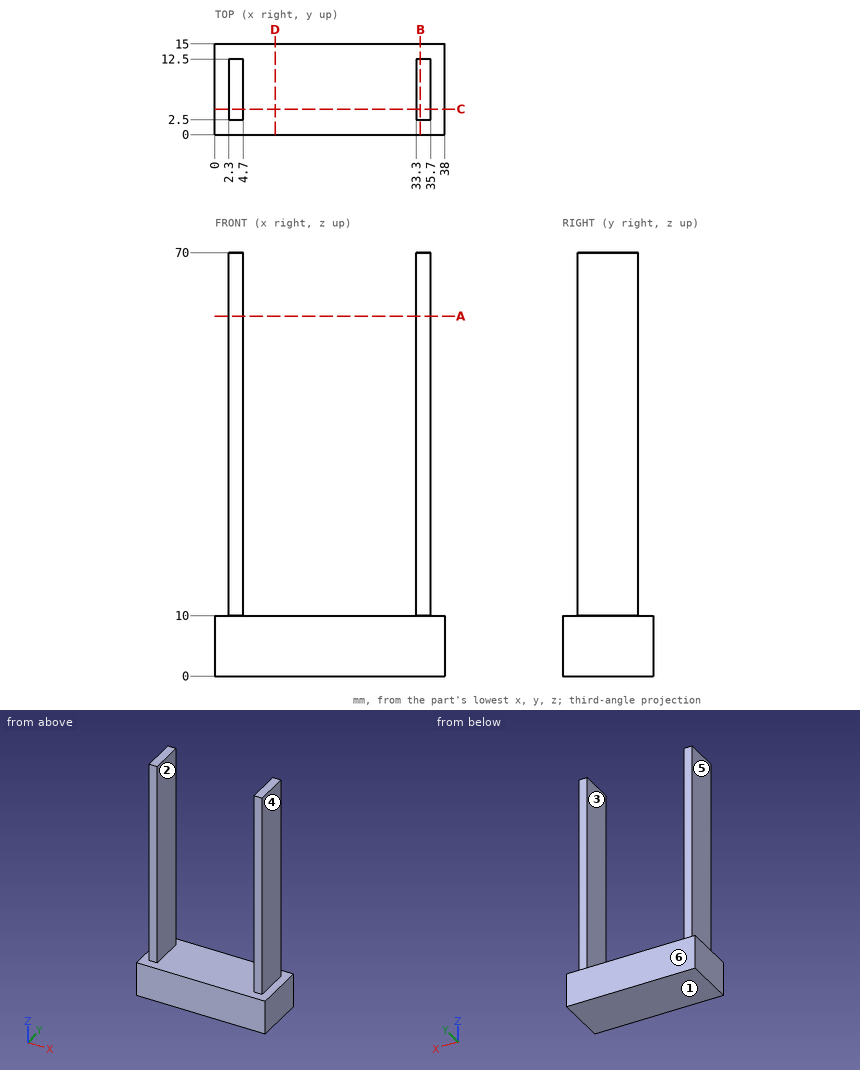
For this review, use the dimensioned drawing (mm, ordinates from the lowest corner) and the shaded views. A direction names the side the tool comes from. Give positions to 0.01 mm unless a question says otherwise; leave off trailing zeros. Order: outer loops, then holes, each group sorted by start corner. A loop starts at its lowest first (then second) coordinate and runs counter-clockwise, first axis right, second up. Notation, with made-up numbers: M 79.25,-15 L 111.25,-15 A10 ccw 111.25,-7 Z; hole C 58,-12 d8. An arc over 180 degrees is marked long. Use one line per item in the form item = value. Start each with the question number.
Item 1: The part is to be moulded in two halves that separate along X. For the marked faces 1, 2, 3 and 4, say which applies: pulls with the +X half, pulls with the -X half, needs draft (parallel to the pull), parting line crosses it, or undercut.
Item 2: For the marked faces 5 and 6, list the 3-axis set-ups (+Z, -Z, +X, -X, +Y, -Y) from which the entire face can be reached by the end or side of a thin tool; tool diameter is ignored.
Item 3: We need section C-C on y = 4.25. Give the boundary of the cut face in (x, z), plus the area to 3 significant figures.
Item 4: We need section A-A on z = 59.5. Give the boundary of the cut face in (x, y).
Item 5: We need section D-D on x = 10. Give the boundary of the cut face in (y, z).
Item 6: We need section B-B on x = 34. Give the boundary of the cut face in (y, z), plus the area to 3 significant figures.
Item 7: To check wall thickness, follow line 1 along X through (y, z) = (8.75, 62); line 2 along Z through (x, y) = (23, 9.5); line 3 along Y through (x, z) = (34, 33.5). State the ranges of each line that lie inside material, in increasing order. Write a range as from..to.
Item 8: Insertion check: pin 1 Ø3 at (y, z) = (9.5, 34) entering from +X; pin 2 Ø1.2 at (x, z) = (34.5, 47) entering from -Y; pin 3 Ø2.5 at (x, z) = (34.5, 31) entering from +Y. Each pin has a flat end and moves straight along its axis. Give the tip position at first contact, or say it passes through.
Completed:
q1.face_1 = needs draft
q1.face_2 = undercut
q1.face_3 = undercut
q1.face_4 = pulls with the +X half
q2.face_5 = +Z, -X, +Y, -Y
q2.face_6 = +Z, -Z, +X, -X, +Y
q3.outline = M 0,0 L 38,0 L 38,10 L 35.7,10 L 35.7,70 L 33.3,70 L 33.3,10 L 4.7,10 L 4.7,70 L 2.3,70 L 2.3,10 L 0,10 Z
q3.area = 668 mm²
q4.outline = M 2.3,2.5 L 4.7,2.5 L 4.7,12.5 L 2.3,12.5 Z; M 33.3,2.5 L 35.7,2.5 L 35.7,12.5 L 33.3,12.5 Z
q5.outline = M 0,0 L 15,0 L 15,10 L 0,10 Z
q6.outline = M 0,0 L 15,0 L 15,10 L 12.5,10 L 12.5,70 L 2.5,70 L 2.5,10 L 0,10 Z
q6.area = 750 mm²
q7.line_1 = 2.3..4.7, 33.3..35.7
q7.line_2 = 0..10
q7.line_3 = 2.5..12.5
q8.pin_1 = 35.7
q8.pin_2 = 2.5
q8.pin_3 = 12.5
